from build123d import *

# Parameters (mm, degrees)
BOSS_EXTRUDE1_DEPTH      = 8.5
BOSS_EXTRUDE1_DEPTH_BACK = 4
SKETCH3_W                = 40
SKETCH3_H                = 3.5
CUT_EXTRUDE1_DEPTH       = 10
BOSS_EXTRUDE2_DEPTH      = 3
SKETCH5_R                = 2.5
BOSS_EXTRUDE3_DEPTH      = 5
SKETCH6_W                = 4
SKETCH6_H                = 2.2
BOSS_EXTRUDE4_DEPTH      = 4


with BuildPart() as part:
    # Sketch1 → Boss-Extrude1 (new body, two sides)
    with BuildSketch(Plane.XY) as boss_extrude1_sk:
        Polygon((0, 0), (0, 65), (35, 65), (35, 55), (15, 55), (15, 15), (35, 15), (35, 0), align=None)
    extrude(amount=BOSS_EXTRUDE1_DEPTH)
    extrude(boss_extrude1_sk.sketch, amount=-BOSS_EXTRUDE1_DEPTH_BACK)

    # Sketch3 → Cut-Extrude1 (cut)
    with BuildSketch(Plane(origin=(0, 65, 0), x_dir=(1, 0, 0), z_dir=(0, 1, 0))):
        with Locations((35, -6.75)):
            Rectangle(SKETCH3_W, SKETCH3_H)
    extrude(amount=-CUT_EXTRUDE1_DEPTH, mode=Mode.SUBTRACT)

    # Sketch4 → Boss-Extrude2 (add)
    with BuildSketch(Plane.XY.offset(8.5)):
        Polygon((35, 0), (0, 0), (0, 65), (35, 65), (35, 52), (18, 52), (18, 18), (35, 18), align=None)
    extrude(amount=BOSS_EXTRUDE2_DEPTH)

    # Sketch5 → Boss-Extrude3 (add)
    with BuildSketch(Plane(origin=(35, 0, 0), x_dir=(0, 0, -1), z_dir=(1, 0, 0))):
        with Locations((-1, 10)):
            Circle(SKETCH5_R)
    extrude(amount=BOSS_EXTRUDE3_DEPTH)

    # Sketch6 → Boss-Extrude4 (add)
    with BuildSketch(Plane(origin=(15, 0, 0), x_dir=(0, 0, -1), z_dir=(1, 0, 0))):
        with Locations((2, 52.2)):
            Rectangle(SKETCH6_W, SKETCH6_H)
        with Locations((2, 17.8)):
            Rectangle(SKETCH6_W, SKETCH6_H)
    extrude(amount=BOSS_EXTRUDE4_DEPTH)


solid = part.part
CAD build for the part. Positions are in the model's coordinates, mm. A direction names the side the tool comes from. Round coordinates to 2 decimals unless told otherwise and drop trailing zeros. Order: outer loops, then holes, each group sorted by start corner. A loop starts at its lowest first (then second) coordinate and runs counter-clockwise, first axis right, second up. Notation, with made-up numbers: M -22.5,72 L 20.5,72 A14 ccw 20.5,92 Z; hole C -17.75,-0.75 d4. An arc over 180 degrees is marked long. Use one line per item in the form item = value.
Q1. Saw through at D-D on y = 44. Give the cut face in (x, z), then the cut area to 4 significant figures.
Recorded:
outline = M 0,-4 L 15,-4 L 15,8.5 L 18,8.5 L 18,11.5 L 0,11.5 Z
area = 241.5 mm^2
Q2. Flat gauge pins, fed straight in: P1, Ø3.5, axis at y = 34, z = 10, coming from the +X side; P2, Ø1.5, axis at x = 29, z = 10, coming from the -Y side; P3, Ø12, axis at x = 22.5, y = 32.5, coming from the -Z side; P4, Ø1.1, axis at y = 17.5, z = -2, coming from the +X side. Where does each tip first touch, or does it go through?
Recorded:
P1 = 18
P2 = 0
P3 = 8.5
P4 = 19
Q3. Two-plate mould, pull along Y, no slides. Class faces 6 (the flat face through (18, 0, 4)), 7 (the flat face through (17, 52, 0)), 8 (the flat face through (17.6, 43.8, 8.5)): +Y half, -Y half, draft (parallel to the pull), parting line (faces both ways), or undercut.
Recorded:
face_6 = -Y half
face_7 = undercut
face_8 = draft
Q4. Which spindle directions (+Z, -Z, +X, -X, +Y, -Y) get a long thin tool onto all of the face, cutting with end or side? Do faces 1 (the flat face through (35, 60, 1)), 2 (the flat face through (40, 10, 1)), 3 (the flat face through (17, 53.3, -2)), 4 (the flat face through (17, 18, 0)), 5 (the flat face through (17, 65, 4)). Say none if no direction does.
Recorded:
face_1 = +Z, -Z, +X, +Y
face_2 = +Z, -Z, +X, +Y, -Y
face_3 = -Z, +X
face_4 = +X
face_5 = +Z, -Z, +X, -X, +Y
Q5. Saw through at A-A on x = 25. Give the cut face in (y, z).
Recorded:
outline = M 0,-4 L 15,-4 L 15,8.5 L 18,8.5 L 18,11.5 L 0,11.5 Z; M 52,8.5 L 65,8.5 L 65,11.5 L 52,11.5 Z; M 55,-4 L 65,-4 L 65,5 L 55,5 Z
Q6. Saw through at B-B on y = 10. Give the cut face in (x, z), then the cut area to 4 significant figures.
Recorded:
outline = M 0,-4 L 35,-4 L 35,-1.5 L 40,-1.5 L 40,3.5 L 35,3.5 L 35,11.5 L 0,11.5 Z
area = 567.5 mm^2
Q7. Saw through at C-C on z = 4.25. Give the cut face in (x, y).
Recorded:
outline = M 0,0 L 35,0 L 35,15 L 15,15 L 15,55 L 35,55 L 35,65 L 0,65 Z
Q8. Probe L1, parallel to Y at x = 28, z = 0.25; L2, parallel to Y at x = 17.5, z = -3; L3, parallel to Z at x = 17.5, y = 58.5. List the from-to ranges inside material, lowest first.
Recorded:
L1 = 0 to 15, 55 to 65
L2 = 0 to 15, 16.7 to 18.9, 51.1 to 53.3, 55 to 65
L3 = -4 to 5, 8.5 to 11.5
